The listing builds one solid part. Answer for the finished solid, in the listing's coordinates (mm). Face numbers are marked on the shaded views. Coordinates: 2 decimals unless noted, no trailing zeros. Order: outer loops, then holes, each group sorted by start corner. A loop starts at its lowest first (then second) coordinate and runs counter-clockwise, first axis right, second up. Notation, with made-up numbers: (10.25, -23) -> (36.25, -23) arc R22 ccw to (36.25, -1) -> close; hole circle Ø3 at (75, 67). An arc over 180 degrees is marked (long way). Write item = value, one per line.
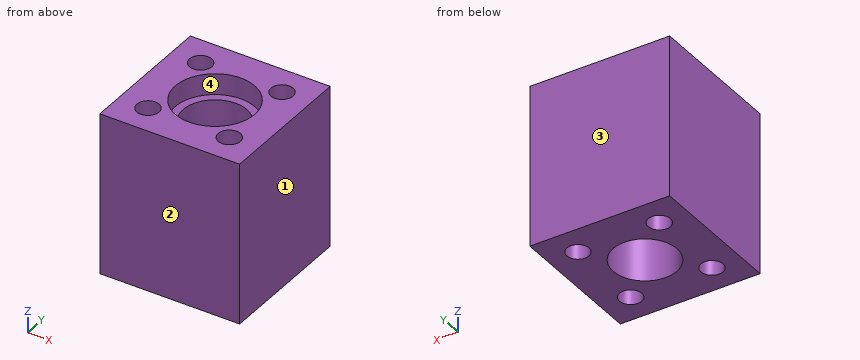
from build123d import *

# Parameters (mm, degrees)
F0_W     = 4.6
F0_H     = 4.6
F0_R     = 6.25
F1_DEPTH = 25.4
F0_R_2   = 5
F2_DEPTH = 22.1
F3_D     = 3.5


with BuildPart() as f1:
    # F0 (on Top) → F1 (new body)
    with BuildSketch(Plane.XY):
        with Locations((8.7, -8.7)):
            Rectangle(F0_W, F0_H)
        Polygon((-6.4, -11), (6.4, -11), (6.4, -6.4), (11, -6.4), (11, 6.4), (6.4, 6.4), (6.4, 11), (-6.4, 11), (-6.4, 6.4), (-11, 6.4), (-11, -6.4), (-6.4, -6.4), align=None)
        Circle(F0_R, mode=Mode.SUBTRACT)
        with Locations((-8.7, -8.7)):
            Rectangle(F0_W, F0_H)
        with Locations((8.7, 8.7)):
            Rectangle(F0_W, F0_H)
        with Locations((-8.7, 8.7)):
            Rectangle(F0_W, F0_H)
    extrude(amount=F1_DEPTH)

    # F0 (on Top) → F2 (join)
    with BuildSketch(Plane.XY):
        Circle(F0_R)
        Circle(F0_R_2, mode=Mode.SUBTRACT)
    extrude(amount=F2_DEPTH)

    # F3 (through all)
    with Locations(Plane(origin=(0, 0, 0), x_dir=(1, 0, 0), z_dir=(0, 0, -1))):
        with Locations((-6.4, -6.4), (-6.4, 6.4), (6.4, -6.4), (6.4, 6.4)):
            Hole(F3_D / 2)


solid = f1.part
Q1. This flat-tipped pin is pushed along its axis until it touches: pin 1 Ø2 at (x, y) = (6.4, -6.4) entering from +Z. Where does it stop, or does it pass through?
The answers:
pin_1 = through
Q2. Section A-A, the plane z = 19.75 is taken. Give the vertices of the cut face in (x, y).
The answers:
outline = (-11, -11) -> (11, -11) -> (11, 11) -> (-11, 11) -> close; hole circle Ø3.5 at (-6.4, -6.4); hole circle Ø3.5 at (-6.4, 6.4); hole circle Ø10 at (0, 0); hole circle Ø3.5 at (6.4, -6.4); hole circle Ø3.5 at (6.4, 6.4)
Q3. The mould has two halves that part along Y. Classify the marked faces 1, 2, 3 and 4: released by +Y, released by -Y, zero draft, split by the parting line, or undercut.
The answers:
face_1 = zero draft
face_2 = released by -Y
face_3 = released by +Y
face_4 = undercut
Q4. Section D-D, the plane z = 23 is taken. Give the vertices of the cut face in (x, y).
The answers:
outline = (-11, -11) -> (11, -11) -> (11, 11) -> (-11, 11) -> close; hole circle Ø3.5 at (-6.4, -6.4); hole circle Ø3.5 at (-6.4, 6.4); hole circle Ø12.5 at (0, 0); hole circle Ø3.5 at (6.4, -6.4); hole circle Ø3.5 at (6.4, 6.4)
Q5. Find the intervals of material crossed by line 1 along Y through (x, z) = (-6.4, 13.25); line 2 along Y through (x, z) = (0, 11.75), in increasing order.
The answers:
line_1 = -11 to -8.15, -4.65 to 4.65, 8.15 to 11
line_2 = -11 to -5, 5 to 11
Q6. Section C-C, the plane y = -5.5 is taken. Give the vertices of the cut face in (x, z), plus the area to 3 significant figures.
The answers:
outline = (-11, 0) -> (-7.9, 0) -> (-7.9, 25.4) -> (-11, 25.4) -> close; (-4.9, 0) -> (4.9, 0) -> (4.9, 25.4) -> (2.97, 25.4) -> (2.97, 22.1) -> (-2.97, 22.1) -> (-2.97, 25.4) -> (-4.9, 25.4) -> close; (7.9, 0) -> (11, 0) -> (11, 25.4) -> (7.9, 25.4) -> close
area = 387 mm2
Q7. Section B-B, the plane x = 0 is taken. Give the vertices of the cut face in (y, z), plus the area to 3 significant figures.
The answers:
outline = (-11, 0) -> (-5, 0) -> (-5, 22.1) -> (-6.25, 22.1) -> (-6.25, 25.4) -> (-11, 25.4) -> close; (5, 0) -> (11, 0) -> (11, 25.4) -> (6.25, 25.4) -> (6.25, 22.1) -> (5, 22.1) -> close
area = 297 mm2
